For this review, take the finished solid that the model builds, in its own axes (mm). A direction names the side the tool comes from. Round coordinates to 2 decimals unless told otherwise and drop trailing zeros. Write each loop counter-clockwise with the first axis right and the second up, starting at its lowest first coordinate (ties: lowest second). Pieces come first, ordered by that corner, then holes. Notation, with made-up numbers: (-31.75, 13) - (-11.75, 13) arc R12 ccw to (-11.75, 20) - close; hole circle Ø7 at (18, 11). An arc over 180 degrees is marked (long way). One line per item, written item: value. Start each with the question number.
Q1. For probe 1 along X at (y, z) = (6.75, 8); probe 2 along Z at (x, y) = (8.5, 1.5), list the stretches that pass through material, from the lowest coordinate up.
Q2. Clearance check with flat-ended pins moving along their axes: pin 1 Ø2 at (x, y) = (5.5, 9.5) entering from +Z; pin 2 Ø4 at (x, z) = (9, 14) entering from +Y. State where each tip first meets the part, or that it passes through.
Q3. Add section B-B on z = 12.25. Write out the cut boundary in (x, y), and give its area (3 significant figures).
Q4. Add section D-D on y = 2. Write out the cut boundary in (x, z), and give its area (3 significant figures).
Q5. Mouldability with a two-part tool opening along Y and no side actions: class faces 1 (the face through (11.5, 12, 2)), 2 (the face through (9, 2, 15)), 3 (the face through (17, 11, 10)) as +Y half, -Y half, draft (parallel to the pull), parting line (faces both ways), or undercut.
Q6. Add section C-C on x = 9.5. Write out the cut boundary in (y, z).
Q7. Tool access review of faces 4 (the face through (9, 9, 2)), 5 (the face through (9, 2, 9)), 6 (the face through (12, 11, 3)): name each direction out of +Z, -Z, +X, -X, +Y, -Y from which nothing blocks a thin tool from reaching the whole face with its end or side.
Q8. Add section A-A on y = 14.5. Write out the cut boundary in (x, z).
```python
from build123d import *

# Parameters (mm, degrees)
SKETCH1_W          = 18
SKETCH1_H          = 18
EXTRUDE1_DEPTH     = 3
SKETCH2_W          = 18
SKETCH2_H          = 3
EXTRUDE2_DEPTH     = 15
EXTRUDE3_DEPTH     = 2
EXTRUDE4_DEPTH     = 2
CUT_EXTRUDE1_REACH = 5
SKETCH7_W          = 5
SKETCH7_H          = 6
CUT_EXTRUDE2_REACH = 5
SKETCH8_W          = 5
SKETCH8_H          = 6


with BuildPart() as part:
    # Sketch1 → Extrude1 (new body)
    with BuildSketch(Plane.XY):
        with Locations((9, 9)):
            Rectangle(SKETCH1_W, SKETCH1_H)
    extrude(amount=EXTRUDE1_DEPTH)

    # Sketch2 → Extrude2 (add)
    with BuildSketch(Plane.XY.offset(3)):
        with Locations((9, 1.5)):
            Rectangle(SKETCH2_W, SKETCH2_H)
    extrude(amount=EXTRUDE2_DEPTH)

    # Sketch5 → Extrude3 (add)
    with BuildSketch(Plane(origin=(18, 0, 0), x_dir=(0, 0, -1), z_dir=(1, 0, 0))):
        Polygon((-3, 18), (-18, 3), (-3, 3), align=None)
    extrude(amount=-EXTRUDE3_DEPTH)

    # Sketch6 → Extrude4 (add)
    with BuildSketch(Plane.ZY):
        Polygon((3, 18), (18, 3), (3, 3), align=None)
    extrude(amount=-EXTRUDE4_DEPTH)

    # Sketch7 → Cut-Extrude1 (cut, up to next)
    with BuildSketch(Plane(origin=(0, 3, 0), x_dir=(1, 0, 0), z_dir=(0, 1, 0)), mode=Mode.PRIVATE) as cut_extrude1_sk1:
        with Locations((9, -12)):
            Rectangle(SKETCH7_W, SKETCH7_H)
    cut_extrude1_tool1 = extrude(cut_extrude1_sk1.sketch, amount=-CUT_EXTRUDE1_REACH, mode=Mode.PRIVATE) & part.part
    add(cut_extrude1_tool1.solids().sort_by_distance((9, 3, 12))[0], mode=Mode.SUBTRACT)

    # Sketch8 → Cut-Extrude2 (cut, up to next)
    with BuildSketch(Plane(origin=(0, 0, 3), x_dir=(-1, 0, 0), z_dir=(0, 0, 1)), mode=Mode.PRIVATE) as cut_extrude2_sk1:
        with Locations((-9, -12)):
            Rectangle(SKETCH8_W, SKETCH8_H)
    cut_extrude2_tool1 = extrude(cut_extrude2_sk1.sketch, amount=-CUT_EXTRUDE2_REACH, mode=Mode.PRIVATE) & part.part
    add(cut_extrude2_tool1.solids().sort_by_distance((9, 12, 3))[0], mode=Mode.SUBTRACT)


solid = part.part
```
Result set:
1. probe 1: x = 0 to 2, 16 to 18
1. probe 2: z = 0 to 9, 15 to 18
2. pin 1: stops at z = 3
2. pin 2: stops at y = 3
3. outline: (0, 0) - (6.5, 0) - (6.5, 3) - (2, 3) - (2, 8.75) - (0, 8.75) - close; (11.5, 0) - (18, 0) - (18, 8.75) - (16, 8.75) - (16, 3) - (11.5, 3) - close
3. area: 62.0 mm^2
4. outline: (0, 0) - (18, 0) - (18, 18) - (0, 18) - close; hole (6.5, 9) - (11.5, 9) - (11.5, 15) - (6.5, 15) - close
4. area: 294 mm^2
5. face 1: undercut
5. face 2: draft
5. face 3: +Y half
6. outline: (0, 0) - (9, 0) - (9, 3) - (3, 3) - (3, 9) - (0, 9) - close; (0, 15) - (3, 15) - (3, 18) - (0, 18) - close; (15, 0) - (18, 0) - (18, 3) - (15, 3) - close
7. face 4: +Z, -Z
7. face 5: +Y, -Y
7. face 6: +Z, +Y
8. outline: (0, 0) - (6.5, 0) - (6.5, 3) - (2, 3) - (2, 6.5) - (0, 6.5) - close; (11.5, 0) - (18, 0) - (18, 6.5) - (16, 6.5) - (16, 3) - (11.5, 3) - close
